Input: part model. Units: mm. Frame: model coordinates. Coordinates: 2 decimals unless noted, no trailing zeros. Order: outer loops, then holes, each group sorted by start corner. A loop starts at its lowest first (then second) coordinate and runs counter-clockwise, first axis right, second up. Notation, with made-up numbers: M 33.5,69.25 L 63.5,69.25 A19 ccw 63.5,82.25 Z; hole C 38,78.25 d7. An arc over 180 degrees is marked long. Answer in a Markdown table with one row per item.
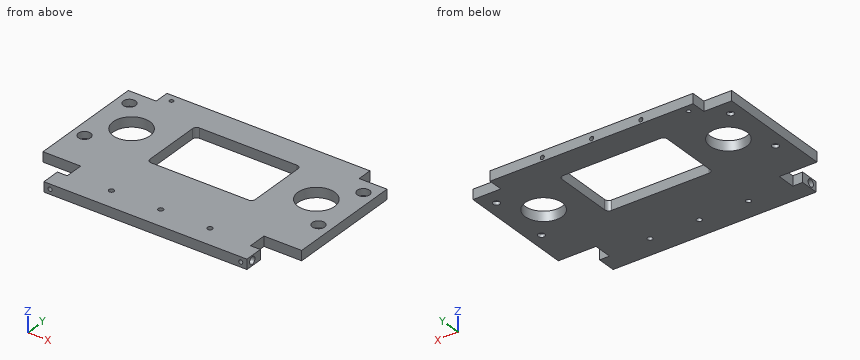
from build123d import *

# Parameters (mm, degrees)
SKETCH_1_W                   = 210
SKETCH_1_H                   = 75
EXTRUDE_1_DEPTH              = 8
CUT_EXTRUDE_1_DEPTH          = 9
HOLE_WIZARD_M5_1_D           = 5.5
HOLE_WIZARD_M5_1_DEPTH       = 10.1
HOLE_WIZARD_M5_1_CBORE_D     = 10
HOLE_WIZARD_M5_1_CBORE_DEPTH = 5.4
HOLE_WIZARD_M5_1_TIP         = 1.652366702
SKETCH_5_R                   = 15
CUT_EXTRUDE_2_DEPTH          = 13
SKETCH_6_W                   = 210
SKETCH_6_H                   = 8
EXTRUDE_2_DEPTH              = 50
SKETCH_7_W                   = 22.6
SKETCH_7_H                   = 30
CUT_EXTRUDE_3_DEPTH          = 20
SKETCH_9_R                   = 3
CUT_EXTRUDE_5_DEPTH          = 8
SKETCH_12_W                  = 164.8
SKETCH_12_H                  = 8
EXTRUDE_3_DEPTH              = 12
SKETCH_13_W                  = 8
SKETCH_13_H                  = 15
CUT_EXTRUDE_6_DEPTH          = 9
HOLE_WIZARD_M4_1_D           = 3.3
HOLE_WIZARD_M4_1_DEPTH       = 5
HOLE_WIZARD_M4_1_TIP         = 0.991420021
HOLE_WIZARD_M4_2_D           = 3.3
HOLE_WIZARD_M4_2_DEPTH       = 10.1
HOLE_WIZARD_M4_2_TIP         = 0.991420021
HOLE_WIZARD_M5_1_2_D         = 4.2
HOLE_WIZARD_M5_1_2_DEPTH     = 8
HOLE_WIZARD_M5_1_2_TIP       = 1.2618073
HOLE_WIZARD_M4_3_D           = 3.3
HOLE_WIZARD_M4_3_DEPTH       = 6
HOLE_WIZARD_M4_3_TIP         = 0.991420021


with BuildPart() as part:
    # 草图1 → 凸台-拉伸1 (new body)
    with BuildSketch(Plane.XY):
        with Locations((105, 37.5)):
            Rectangle(SKETCH_1_W, SKETCH_1_H)
    extrude(amount=EXTRUDE_1_DEPTH)

    # 草图2 → 切除-拉伸1 (cut, through all)
    with BuildSketch(Plane.XY.offset(8)):
        with BuildLine():
            Line((144.62, 64.5), (65.38, 64.5))
            ThreePointArc((65.38, 64.5), (63.131400436, 63.568599564), (62.2, 61.32))
            Line((62.2, 61.32), (62.2, 13.68))
            ThreePointArc((62.2, 13.68), (63.131400436, 11.431400436), (65.38, 10.5))
            Line((65.38, 10.5), (144.62, 10.5))
            ThreePointArc((144.62, 10.5), (146.868599564, 11.431400436), (147.8, 13.68))
            Line((147.8, 13.68), (147.8, 61.32))
            ThreePointArc((147.8, 61.32), (146.868599564, 63.568599564), (144.62, 64.5))
        make_face()
    extrude(amount=-CUT_EXTRUDE_1_DEPTH, mode=Mode.SUBTRACT)

    # Hole Wizard M5 _1
    with Locations(Plane.XY.offset(8)):
        with Locations((10, 62.5), (10, 12.5), (200, 62.5), (200, 12.5)):
            CounterBoreHole(HOLE_WIZARD_M5_1_D / 2, HOLE_WIZARD_M5_1_CBORE_D / 2, HOLE_WIZARD_M5_1_CBORE_DEPTH, depth=HOLE_WIZARD_M5_1_DEPTH)
            with Locations((0, 0, -(HOLE_WIZARD_M5_1_DEPTH + HOLE_WIZARD_M5_1_TIP / 2))):  # 118° drill point
                Cone(0, HOLE_WIZARD_M5_1_D / 2, HOLE_WIZARD_M5_1_TIP, mode=Mode.SUBTRACT)

    # 草图5 → 切除-拉伸2 (cut)
    with BuildSketch(Plane.XY.offset(8)):
        with Locations((30, 37.5)):
            Circle(SKETCH_5_R)
        with Locations((180, 37.5)):
            Circle(SKETCH_5_R)
    extrude(amount=-CUT_EXTRUDE_2_DEPTH, mode=Mode.SUBTRACT)

    # 草图6 → 凸台-拉伸2 (add)
    with BuildSketch(Plane.XZ):
        with Locations((105, 4)):
            Rectangle(SKETCH_6_W, SKETCH_6_H)
    extrude(amount=EXTRUDE_2_DEPTH)

    # 草图7 → 切除-拉伸3 (cut)
    with BuildSketch(Plane.XY.offset(8)):
        with Locations((11.3, -35)):
            Rectangle(SKETCH_7_W, SKETCH_7_H)
        with Locations((198.7, -35)):
            Rectangle(SKETCH_7_W, SKETCH_7_H)
    extrude(amount=-CUT_EXTRUDE_3_DEPTH, mode=Mode.SUBTRACT)

    # 草图9 → 切除-拉伸5 (cut)
    with BuildSketch(Plane.ZY.offset(-22.6)):
        with Locations((3.9960026, -44.027952664)):
            Circle(SKETCH_9_R)
    cut_extrude_5 = extrude(amount=-CUT_EXTRUDE_5_DEPTH, mode=Mode.SUBTRACT)

    # 镜向1: 切除-拉伸5 across plane
    add(cut_extrude_5.mirror(Plane.ZY.offset(-105)), mode=Mode.SUBTRACT)

    # 草图12 → 凸台-拉伸3 (add)
    with BuildSketch(Plane(origin=(0, 75, 0), x_dir=(1, 0, 0), z_dir=(0, 1, 0))):
        with Locations((105, -4)):
            Rectangle(SKETCH_12_W, SKETCH_12_H)
    extrude(amount=EXTRUDE_3_DEPTH)

    # 草图13 → 切除-拉伸6 (cut, through all)
    with BuildSketch(Plane.XY.offset(8)):
        with Locations((26.6, -27.5)):
            Rectangle(SKETCH_13_W, SKETCH_13_H)
        with Locations((183.4, -27.5)):
            Rectangle(SKETCH_13_W, SKETCH_13_H)
    extrude(amount=-CUT_EXTRUDE_6_DEPTH, mode=Mode.SUBTRACT)

    # M4 螺纹孔1
    with Locations(Plane(origin=(0, -50, 0), x_dir=(-1, 0, 0), z_dir=(0, -1, 0))):
        with Locations((-27.6, -4.002197451), (-182.4, -4.002197451)):
            Hole(HOLE_WIZARD_M4_1_D / 2, depth=HOLE_WIZARD_M4_1_DEPTH)
            with Locations((0, 0, -(HOLE_WIZARD_M4_1_DEPTH + HOLE_WIZARD_M4_1_TIP / 2))):  # 118° drill point
                Cone(0, HOLE_WIZARD_M4_1_D / 2, HOLE_WIZARD_M4_1_TIP, mode=Mode.SUBTRACT)

    # M4 螺纹孔2
    with Locations(Plane(origin=(0, 0, 0), x_dir=(-1, 0, 0), z_dir=(0, 0, -1))):
        with Locations((-30.6, 81)):
            Hole(HOLE_WIZARD_M4_2_D / 2, depth=HOLE_WIZARD_M4_2_DEPTH)
            with Locations((0, 0, -(HOLE_WIZARD_M4_2_DEPTH + HOLE_WIZARD_M4_2_TIP / 2))):  # 118° drill point
                Cone(0, HOLE_WIZARD_M4_2_D / 2, HOLE_WIZARD_M4_2_TIP, mode=Mode.SUBTRACT)

    # Hole Wizard M5 _1 2
    with Locations(Plane.XY.offset(8)):
        with Locations((65, -32.942976998), (105, -32.942976998), (145, -32.942976998)):
            Hole(HOLE_WIZARD_M5_1_2_D / 2, depth=HOLE_WIZARD_M5_1_2_DEPTH)
            with Locations((0, 0, -(HOLE_WIZARD_M5_1_2_DEPTH + HOLE_WIZARD_M5_1_2_TIP / 2))):  # 118° drill point
                Cone(0, HOLE_WIZARD_M5_1_2_D / 2, HOLE_WIZARD_M5_1_2_TIP, mode=Mode.SUBTRACT)

    # M4 螺纹孔3
    with Locations(Plane(origin=(0, 87, 0), x_dir=(1, 0, 0), z_dir=(0, 1, 0))):
        with Locations((145, -3), (105, -3), (65, -3)):
            Hole(HOLE_WIZARD_M4_3_D / 2, depth=HOLE_WIZARD_M4_3_DEPTH)
            with Locations((0, 0, -(HOLE_WIZARD_M4_3_DEPTH + HOLE_WIZARD_M4_3_TIP / 2))):  # 118° drill point
                Cone(0, HOLE_WIZARD_M4_3_D / 2, HOLE_WIZARD_M4_3_TIP, mode=Mode.SUBTRACT)


solid = part.part
1) Cut plane B-B, the plane x = 10. Output: boundary loops of the cut face in (y, z).
Resolved:
| item | result |
|---|---|
| outline | M -20,0 L 9.75,0 L 9.75,2.6 L 7.5,2.6 L 7.5,8 L -20,8 Z; M 15.25,0 L 59.75,0 L 59.75,2.6 L 57.5,2.6 L 57.5,8 L 17.5,8 L 17.5,2.6 L 15.25,2.6 Z; M 65.25,0 L 75,0 L 75,8 L 67.5,8 L 67.5,2.6 L 65.25,2.6 Z |
2) Cut plane A-A, the plane x = 121.5. Output: boundary loops of the cut face in (y, z), and give its area (3 significant figures).
Resolved:
| item | result |
|---|---|
| outline | M -50,0 L 10.5,0 L 10.5,8 L -50,8 Z; M 64.5,0 L 87,0 L 87,8 L 64.5,8 Z |
| area | 664 mm2 |
3) Cut plane C-C, the plane x = 38. Output: boundary loops of the cut face in (y, z), and give its area (3 significant figures).
Resolved:
| item | result |
|---|---|
| outline | M -50,0 L 24.81,0 L 24.81,8 L -50,8 Z; M 50.19,0 L 87,0 L 87,8 L 50.19,8 Z |
| area | 893 mm2 |
4) Material intervals for probe 1 along Y at (x, z) = (31, 6.5); probe 2 along X at (y, z) = (-33, 1); probe 3 along Y at (x, z) = (200, 6.85), sorted ascending.
Resolved:
| item | result |
|---|---|
| probe 1 | y = -50 to 22.53, 52.47 to 79.4, 82.6 to 87 |
| probe 2 | x = 30.6 to 62.9, 67.1 to 102.9, 107.1 to 142.9, 147.1 to 179.4 |
| probe 3 | y = -20 to 7.5, 17.5 to 57.5, 67.5 to 75 |
5) Contact query for flat-ended pins moving along their axis: pin 1 (3 mm diameter, centred on x = 11.5, y = 62, fed in from +Z); pin 2 (4 mm diameter, centred on y = -28.5, z = 2.5, fed in from +X); pin 3 (2.5 mm diameter, centred on x = 12.5, z = 5, fed in from -Y). Output: stop coordinate, or through.
Resolved:
| item | result |
|---|---|
| pin 1 | stops at z = 2.6 |
| pin 2 | stops at x = 179.4 |
| pin 3 | stops at y = -20 |
